Part model, mm, in its own coordinate system. Coordinates: 2 decimals unless noted, no trailing zeros. Write each loop counter-clockwise with the first axis right and the second up, starting at its lowest first coordinate (ties: lowest second). Pieces come first, ordered by that corner, then holes. Notation, with made-up numbers: (48.25, -27) -> (52.25, -27) arc R17 ccw to (52.25, -10) -> close; hole circle Ø5 at (61, 84.5). An arc over 180 degrees is marked (long way). Write item = value, one per line.
from build123d import *

# Parameters (mm, degrees)
SALIENTE_EXTRUIR1_DEPTH = 3


with BuildPart() as part:
    # Croquis1 → Saliente-Extruir1 (new body)
    with BuildSketch(Plane(origin=(0, 0, 0), x_dir=(1, 0, 0), z_dir=(0, 1, 0))):
        Polygon((20, 250), (14, 250), (14, 253), (10, 253), (6, 253), (6, 250), (3, 250), (0, 250), (0, 200), (3, 200), (3, 150), (0, 150), (0, 100), (3, 100), (3, 50), (0, 50), (0, 0), (6, 0), (6, -3), (14, -3), (14, 0), (20, 0), (20, 50), (17, 50), (17, 100), (20, 100), (20, 125), (20, 150), (17, 150), (17, 200), (20, 200), align=None)
        Polygon((8.5, 244), (10, 244), (11.5, 244), (11.5, 236), (8.5, 236), align=None, mode=Mode.SUBTRACT)
    extrude(amount=SALIENTE_EXTRUIR1_DEPTH)


solid = part.part
Q1. Probe line 1 (Z direction, x = 1, y = 1.3); line 2 (Z direction, x = 10.75, y = 0.55); line 3 (X direction, y = 1.05, z = -87). List the from-to ranges inside material, lowest first. Write a range as from..to.
Model answer:
line_1 = -250..-200, -150..-100, -50..0
line_2 = -253..-244, -236..3
line_3 = 3..17
Q2. Saw through at B-B on z = -183. Give the cut face in (x, y), and give its area (3 significant figures).
Model answer:
outline = (3, 0) -> (17, 0) -> (17, 3) -> (3, 3) -> close
area = 42.0 mm²
Q3. Pin check, flat tips, straight feed: pin 1 (1.5 mm diameter, centred on x = 1, y = 2, fed in from -Z); pin 2 (0.9 mm diameter, centred on x = 1, y = 1.5, fed in from +Z); pin 3 (1.5 mm diameter, centred on y = 1.5, z = 2, fed in from -X). Stop position of each tip, or through.
Model answer:
pin_1 = -250
pin_2 = 0
pin_3 = 6
